from build123d import *

# Parameters (mm, degrees)
SKETCH1_W           = 180
SKETCH1_H           = 60
SKETCH1_R           = 3
BOSS_EXTRUDE1_DEPTH = 50
SKETCH2_R           = 3
CUT_EXTRUDE1_DEPTH  = 10
FILLET1_R           = 10


with BuildPart() as part:
    # Sketch1 → Boss-Extrude1 (new body)
    with BuildSketch(Plane(origin=(0, 0, 0), x_dir=(1, 0, 0), z_dir=(0, 1, 0))):
        with Locations((90, 30)):
            Rectangle(SKETCH1_W, SKETCH1_H)
        with Locations((20, 30)):
            Circle(SKETCH1_R, mode=Mode.SUBTRACT)
        with Locations((160, 30)):
            Circle(SKETCH1_R, mode=Mode.SUBTRACT)
    extrude(amount=BOSS_EXTRUDE1_DEPTH)

    # Sketch2 → Cut-Extrude1 (cut)
    with BuildSketch(Plane(origin=(180, 0, 0), x_dir=(0, 0, -1), z_dir=(1, 0, 0))):
        with Locations((30, 25)):
            Circle(SKETCH2_R)
    extrude(amount=-CUT_EXTRUDE1_DEPTH, mode=Mode.SUBTRACT)

    # Fillet1
    fillet1_edges = [part.edges().sort_by_distance(p)[0] for p in [
        (0, 25, -60),
        (180, 25, -60),
        (180, 25, 0),
        (0, 25, 0),
    ]]
    fillet(fillet1_edges, radius=FILLET1_R)


solid = part.part
Model file for the job. Use its own axes, mm. A direction names the side the tool comes from. Give positions to 0.01 mm unless a question says otherwise; leave off trailing zeros. Loops run counter-clockwise (first coordinate to the right, second up) from the corner with the lowest first, then second, coordinate; pieces in that order, holes last.
1) Saw through at B-B (z = -30). Write the cut outline in (x, y).
2) Tool access for faces 5 (the flat face through (170, 25, -30)), 6 (the flat face through (89, 25, 0)): list every direction of +Z, -Z, +X, -X, +Y, -Y with a clear straight run to the whole face (end or side of a thin tool).
3) Saw through at C-C (y = 25). Write the cut outline in (x, z).
4) Pull direction Y, two halves, no side cores. Call faces 1 (the cylindrical face through (175, 25, -27)), 2 (the flat face through (0, 25, -30)), 3 (the flat face through (89, 0, -30)), 4 (the flat face through (89, 50, -30)): +Y half, -Y half, draft (parallel to the pull), parting line (faces both ways), or undercut.
5) Wall check: line 1 (X direction, y = 15, z = -30); line 2 (Z direction, x = 20, y = 17); line 3 (X direction, y = 29, z = -31.5). Give the ranges that are in metal, low to high.
6) Saw through at A-A (x = 20). Write the cut outline in (y, z), plus the area to 3 significant figures.
7) Flat gauge pins, fed straight in: pin 1 Ø3 at (y, z) = (25.5, -30) entering from +X; pin 2 Ø5.5 at (x, z) = (20, -30) entering from -Y; pin 3 Ø1 at (y, z) = (34, -7.5) entering from -X; pin 4 Ø4 at (y, z) = (37, -7.5) entering from -X. Where does each tip first touch, or does it go through?
Answer block:
1. outline: (0, 0) - (17, 0) - (17, 50) - (0, 50) - close; (23, 0) - (157, 0) - (157, 50) - (23, 50) - close; (163, 0) - (180, 0) - (180, 22) - (170, 22) - (170, 28) - (180, 28) - (180, 50) - (163, 50) - close
2. face 5: +X
2. face 6: +Z, +X, -X, +Y, -Y
3. outline: (0, -50) arc R10 ccw to (10, -60) - (170, -60) arc R10 ccw to (180, -50) - (180, -33) - (170, -33) - (170, -27) - (180, -27) - (180, -10) arc R10 ccw to (170, 0) - (10, 0) arc R10 ccw to (0, -10) - close; hole circle Ø6 at (20, -30); hole circle Ø6 at (160, -30)
4. face 1: undercut
4. face 2: draft
4. face 3: -Y half
4. face 4: +Y half
5. line 1: x = 0 to 17, 23 to 157, 163 to 180
5. line 2: z = -60 to -33, -27 to 0
5. line 3: x = 0 to 17.4, 22.6 to 157.4, 162.6 to 180
6. outline: (0, -60) - (50, -60) - (50, -33) - (0, -33) - close; (0, -27) - (50, -27) - (50, 0) - (0, 0) - close
6. area: 2,700 mm2
7. pin 1: stops at x = 170
7. pin 2: passes through
7. pin 3: stops at x = 0.2
7. pin 4: stops at x = 0.01
